Build history of the part. All positions in model axes, mm. Give positions to 0.01 mm unless a question says otherwise; leave off trailing zeros. Order: outer loops, then holes, each group sorted by start corner. A loop starts at its lowest first (then second) coordinate and runs counter-clockwise, first axis right, second up. Notation, with made-up numbers: M -16.5,23.5 L 18.5,23.5 A33 cw 18.5,57.5 Z; hole C 84.5,88.25 d1. An arc over 180 degrees is marked long. Answer as CSV lines item,"result".
Autodesk Inventor part; units mm, degrees
ref_plane "YZ Plane" through (0, 0, 0) normal (1, 0, 0) x (0, 1, 0)
ref_plane "XZ Plane" through (0, 0, 0) normal (0, 1, 0) x (-1, 0, 0)
ref_plane "XY Plane" through (0, 0, 0) normal (0, 0, 1) x (1, 0, 0)
sketch "Sketch1" plane through (0, 0, 0) normal (0, 1, 0) x (-1, 0, 0)
  circle A0 centre (0, 0) radius 5
  dimension "d0" = 10
extrude "Extrusion1" add sketch "Sketch1" along normal blind 100 and the other way blind 10
sketch "Sketch2" plane through (0, 0, 0) normal (0, 0, 1) x (1, 0, 0)
  circle A0 centre (0, 0) radius 3.065
  dimension "d5" = 6.13
extrude "Extrusion2" cut sketch "Sketch2" along normal mid plane 100
chamfer "Chamfer1" distance 2 angle 45 2 edges at (5, 100, 0) (5, -10, 0)
properties part number "pendulum"
Item 1: Band-saw the part on B-B (z = 0). Give the cut face in (x, y) (3 decimals), and give its area (3 significant figures).
Geometry says:
outline,"M -5,-8 L -3,-10 L 3,-10 L 5,-8 L 5,98 L 3,100 L -3,100 L -5,98 Z; hole C 0,0 d6.13"
area,"1,060 mm2"
Item 2: Band-saw the part on C-C (y = 49). Give the cut face in (x, z).
Geometry says:
outline,"C 0,0 d10"
Item 3: Band-saw the part on A-A (x = 0). Give the cut face in (y, z) (3 decimals).
Geometry says:
outline,"M -10,-3 L -8,-5 L -3.065,-5 L -3.065,5 L -8,5 L -10,3 Z; M 3.065,-5 L 98,-5 L 100,-3 L 100,3 L 98,5 L 3.065,5 Z"
Item 4: Probe line 1 along Y through (x, z) = (0, 2.25) (3 decimals); line 2 along X through (y, z) = (0, -0.25) (3 decimals); line 3 along X through (y, z) = (-1, -2). List the from-to ranges inside material, lowest first. Write a range as from..to.
Geometry says:
line 1,"y = -10..-3.065, 3.065..100"
line 2,"x = -4.994..-3.065, 3.065..4.994"
line 3,"x = -4.58..-2.9, 2.9..4.58"
Item 5: Drop flat-ended pins along their axis: pin 1 (1.5 mm diameter, centred on x = 1.5, y = 41, fed in from +Z); pin 2 (5 mm diameter, centred on x = -2.5, y = 76, fed in from -Z); pin 3 (1.5 mm diameter, centred on x = -4, y = 76, fed in from +Z). Give the stop position or say it passes through.
Geometry says:
pin 1,"stops at z = 4.94"
pin 2,"stops at z = -5"
pin 3,"stops at z = 3.8"
Item 6: Band-saw the part on D-D (y = 0). Give the cut face in (x, z) (3 decimals), and give its area (3 significant figures).
Geometry says:
outline,"M -3.065,-3.95 L -3.065,3.95 A5 ccw Z; M 3.065,-3.95 A5 ccw 3.065,3.95 Z"
area,"21.3 mm2"
